Work out the finished part from the listing and answer in its coordinate system (mm). Face numbers are marked on the shaded views. A direction names the side the tool comes from. Coordinates: 2 decimals unless noted, no trailing zeros. Write each loop counter-clockwise with the first axis right and the second up, starting at its lowest first coordinate (ties: lowest second). Pieces come first, ordered by that corner, then holes. Notation, with made-up numbers: M 32.25,-4 L 59.25,-4 A7 ccw 59.25,0 Z; hole C 52.25,62.5 d6. An arc over 180 degrees is marked long. Answer as CSV lines item,"result". Start each with the question number.
(1) Find the intervals of material crossed by L1, parallel to Y at x = -56, z = 40; L2, parallel to X at y = -17, z = 59, in increasing order. Write a range as [from, to].
(2) A cutting plane is placed at A-A on z = 94. Give the vertices of the cut face in (x, y), then the cut area to 3 significant figures.
(3) For the marked faces 5 and 6, determine the directions among +Z, -Z, +X, -X, +Y, -Y from which every point of the face is accessible in a straight line to the end or side of a thin tool.
(4) The mould has two halves that part along X. Classify the marked faces 1, 2, 3 and 4: released by +X, released by -X, zero draft, split by the parting line, or undercut.
Autodesk Fusion 360 part; units mm, degrees
sketch "草图2" plane through (0, 0, 0) normal (0, 0, 1) x (1, 0, 0)
  line L0 (68, 55) -> (-68, 55)
  line L1 (-70, 53) -> (-70, -53)
  line L2 (-68, -55) -> (68, -55)
  line L3 (70, -53) -> (70, 53)
  line L4 (70, 55) -> (-70, -55) construction
  line L5 (-70, 55) -> (70, -55) construction
  arc A0 (70, 53) -> (68, 55) centre (68, 53) ccw
  arc A1 (68, -55) -> (70, -53) centre (68, -53) ccw
  arc A2 (-70, -53) -> (-68, -55) centre (-68, -53) ccw
  arc A3 (-68, 55) -> (-70, 53) centre (-68, 53) ccw
  line L6 (-68, -58) -> (68, -58)
  line L7 (73, -53) -> (73, 53)
  line L8 (68, 58) -> (-68, 58)
  line L9 (-73, 53) -> (-73, -53)
  line L10 (-73, 58) -> (73, 58)
  line L11 (73, 58) -> (73, -58)
  line L12 (73, -58) -> (-73, -58)
  line L13 (-73, -58) -> (-73, 58)
  dimension "d11" = 140
  dimension "d12" = 110
  dimension "d14" = 2
  dimension "d15" = 116
  dimension "d16" = 146
extrude "拉伸1" add sketch "草图2" along normal blind 100
fillet "圆角1" radius 3 8 edges at (70, 0, 100) (69.4142, -54.4142, 100) (0, -55, 100) (-69.4142, -54.4142, 100) (-70, 0, 100) (-69.4142, 54.4142, 100) (0, 55, 100) (69.4142, 54.4142, 100)
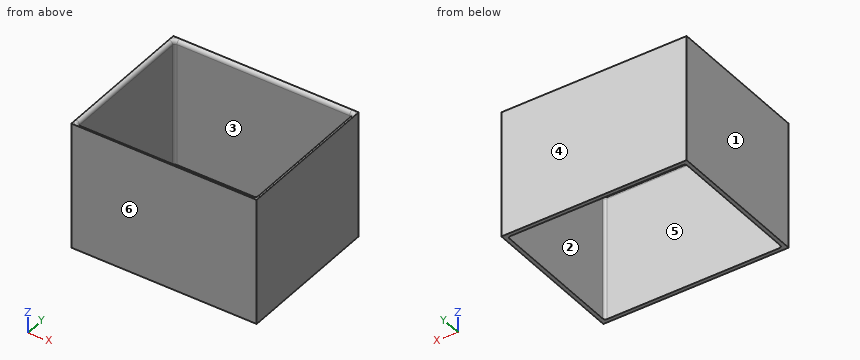
Here are the results:
1,L1,"y = [-58, -55], [55, 58]"
1,L2,"x = [-73, -70], [70, 73]"
2,outline,"M -73,-58 L 73,-58 L 73,58 L -73,58 Z; hole M -70,-53 A2 ccw -68,-55 L 68,-55 A2 ccw 70,-53 L 70,53 A2 ccw 68,55 L -68,55 A2 ccw -70,53 Z"
2,area,"1,540 mm^2"
3,face 5,"+Z, -Z"
3,face 6,"+Z, -Z, +X, -X, -Y"
4,face 1,"released by -X"
4,face 2,"undercut"
4,face 3,"undercut"
4,face 4,"zero draft"
